from build123d import *

# Parameters (mm, degrees)
F4_DEPTH = 25.4
F5_ANGLE = 90
F7_W     = 63.5
F7_H     = 63.5
F8_DEPTH = 88.9


with BuildPart() as f1:
    # F0 (on Front) → F1 (revolve)
    with BuildSketch(Plane.XZ):
        with BuildLine():
            Line((0, 63.5), (0, -63.5))
            ThreePointArc((0, -63.5), (44.9012806053, -44.9012806053), (63.5, 0))
            ThreePointArc((63.5, 0), (44.9012806053, 44.9012806053), (0, 63.5))
        make_face()
    revolve(axis=Axis((0, 0, 5.784236908), (0, 0, 1)))

    # F3 (on offset) → F4 (join)
    with BuildSketch(Plane.XZ.offset(25.4)):
        with BuildLine():
            Line((-63.5, 0), (63.5, 0))
            ThreePointArc((63.5, 0), (0, 63.5), (-63.5, 0))
        make_face()
    extrude(amount=-F4_DEPTH)

    # F4_face (on face) → F5 (revolve)
    with BuildSketch(Plane(origin=(0, -25.4, 38.7624051915), x_dir=(1, 0, 0), z_dir=(0, -1, 0))):
        with BuildLine():
            ThreePointArc((63.5, -38.7624051915), (0, 24.7375948085), (-63.5, -38.7624051915))
            Line((-63.5, -38.7624051915), (-58.1987113259, -38.7624051915))
            ThreePointArc((-58.1987113259, -38.7624051915), (0, 19.4363061344), (58.1987113259, -38.7624051915))
            Line((58.1987113259, -38.7624051915), (63.5, -38.7624051915))
        make_face()
    revolve(axis=Axis((-60.849355663, -25.4, 0), (1, 0, 0)), revolution_arc=F5_ANGLE)

    # F7 (on offset) → F8 (join)
    with BuildSketch(Plane.XZ.offset(88.9)):
        with Locations((-31.75, -31.75)):
            Rectangle(F7_W, F7_H)
        with Locations((31.75, -31.75)):
            Rectangle(F7_W, F7_H)
    extrude(amount=-F8_DEPTH)


solid = f1.part
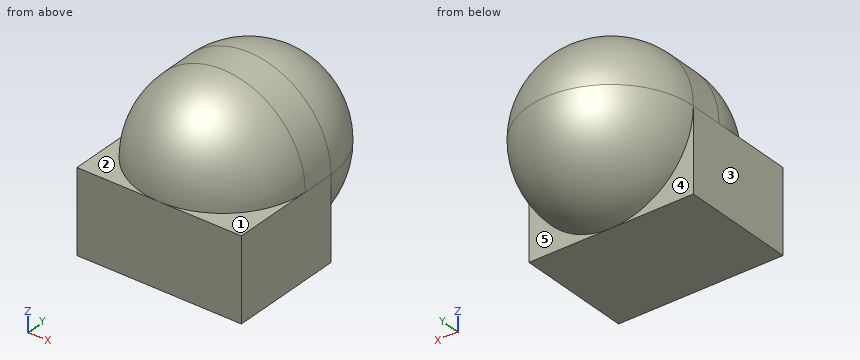
Geometry check sheet. Reference: the model listing, model coordinates, mm. Face numbers are marked on the shaded views. A direction names the side the tool comes from. Round coordinates to 2 decimals unless told otherwise and drop trailing zeros. Order: outer loops, then holes, each group sorted by start corner. A loop starts at its lowest first (then second) coordinate and runs counter-clockwise, first axis right, second up. Notation, with made-up numbers: M 44,82 L 77,82 A5 cw 77,89 Z; hole C -34,-15.75 d6. An arc over 180 degrees is marked long. Write each question's results on one line, items separated by ' | '. Start each with the question number.
1. Cross-section at C-C on z = 41.5. Record the boundary of the cut face in (x, y), plus the area to 3 significant figures.
2. Cross-section at B-B on y = -34.5. Record the boundary of the cut face in (x, z), plus the area to 3 significant figures.
3. Material ranges on L1, parallel to Y at x = -16, z = 47; L2, parallel to Z at x = -42.5, y = -81.5; L3, parallel to Y at x = -56.5, z = -34, recorded low to high. Write a range as from..to.
4. Go/stop test with flat-tipped pins: P1, Ø1.5, axis at x = -13.5, y = 16.5, coming from the -Z side; P2, Ø8, axis at x = 30, z = 44.5, coming from the -Y side; P3, Ø10, axis at x = -38, y = -22, coming from the +Z side. Record where each tip stops, or that it passes through.
5. Cross-section at A-A on x = -6. Record the boundary of the cut face in (y, z).
6. Cross-section at D-D on z = -35.5. Record the boundary of the cut face in (x, y).
7. Set-up check for the marked faces 1, 2, 3, 4 and 5: record each of +Z, -Z, +X, -X, +Y, -Y from which the full face is reachable in a straight line by a thin tool's end or side.
Resolved:
1) outline: M -48.06,-25.4 A48.06 ccw 48.06,-25.4 L 48.06,0 A48.06 ccw -48.06,0 Z; hole M -40.8,-25.4 A40.8 ccw 40.8,-25.4 A48.06 cw Z | area: 8,390 mm2
2) outline: M -63.5,-63.5 L 63.5,-63.5 L 63.5,0 L 62.84,0 A62.84 ccw -62.84,0 L -63.5,0 Z; hole M -57.48,0 L -53.31,0 A53.31 cw 53.31,0 L 57.48,0 A57.48 ccw Z | area: 13,500 mm2
3) L1: -64.99..-55.77, -39.59..39.59 | L2: -63.5..0 | L3: -88.9..0
4) P1: z = -60.08 | P2: y = -64.96 | P3: z = 54.25
5) outline: M -88.9,-63.5 L 0,-63.5 L 0,-63.22 A63.22 ccw 0,63.22 L -25.4,63.22 A63.22 ccw -88.62,0 L -88.9,0 Z; hole M -83.29,0 L -63.22,0 A63.22 cw -25.4,57.89 A57.89 ccw Z
6) outline: M -63.5,-88.9 L 63.5,-88.9 L 63.5,0 L 52.65,0 A52.65 ccw -52.65,0 L -63.5,0 Z
7) face 1: +Z, +X, -Y | face 2: +Z, -X, -Y | face 3: +Z, -Z, -X, +Y, -Y | face 4: -Z, -X, +Y | face 5: -Z, +X, +Y
